from build123d import *

# Parameters (mm, degrees)
SKETCH1_W           = 22
SKETCH1_H           = 112
BOSS_EXTRUDE1_DEPTH = 21
CUT_EXTRUDE1_DEPTH  = 19
FILLET1_START       = -1
FILLET1_DEPTH       = 113
FILLET1_2_DEPTH     = 113
FILLET1_3_DEPTH     = 24
CUT_EXTRUDE11_DEPTH = 116.870617501


with BuildPart() as part:
    # Sketch1 → Boss-Extrude1 (new body)
    with BuildSketch(Plane(origin=(0, 0, 0), x_dir=(1, 0, 0), z_dir=(0, 1, 0))):
        with Locations((11, -56)):
            Rectangle(SKETCH1_W, SKETCH1_H)
    extrude(amount=BOSS_EXTRUDE1_DEPTH)

    # Sketch2 → Cut-Extrude1 (cut)
    with BuildSketch(Plane.XZ):
        Polygon((0, 112), (22, 112), (22, 0), (21, 0), (21, 111), (1, 111), (1, 0), (0, 0), align=None)
    extrude(amount=-CUT_EXTRUDE1_DEPTH, mode=Mode.SUBTRACT)

    # Fillet1: read off the stored shape, not the designer's step
    # Fillet1 outline → Fillet1 (cut)
    with BuildSketch(Plane.XY.offset(FILLET1_START)):
        with BuildLine():
            Line((0, 19), (1, 19))
            ThreePointArc((1, 19), (0.292893219, 19.292893219), (0, 20))
            Line((0, 20), (0, 19))
        make_face()
        with BuildLine():
            ThreePointArc((22, 20), (21.707106781, 19.292893219), (21, 19))
            Line((21, 19), (22, 19))
            Line((22, 19), (22, 20))
        make_face()
    extrude(amount=FILLET1_DEPTH, mode=Mode.SUBTRACT)

    # Fillet1 2 outline → Fillet1 2 (cut)
    with BuildSketch(Plane.XY.offset(FILLET1_START)):
        with BuildLine():
            Line((0, 21), (0, 20))
            ThreePointArc((0, 20), (0.292893219, 20.707106781), (1, 21))
            Line((1, 21), (0, 21))
        make_face()
        with BuildLine():
            Line((22, 21), (21, 21))
            ThreePointArc((21, 21), (21.707106781, 20.707106781), (22, 20))
            Line((22, 20), (22, 21))
        make_face()
    extrude(amount=FILLET1_2_DEPTH, mode=Mode.SUBTRACT)

    # Fillet1 3 outline → Fillet1 3 (cut)
    with BuildSketch(Plane.YZ.offset(FILLET1_START)):
        with BuildLine():
            Line((21, 112), (20, 112))
            ThreePointArc((20, 112), (20.707106781, 111.707106781), (21, 111))
            Line((21, 111), (21, 112))
        make_face()
        with BuildLine():
            ThreePointArc((19, 111), (19.292893219, 111.707106781), (20, 112))
            Line((20, 112), (19, 112))
            Line((19, 112), (19, 111))
        make_face()
    extrude(amount=FILLET1_3_DEPTH, mode=Mode.SUBTRACT)

    # Sketch11 → Cut-Extrude11 (cut, through all)
    with BuildSketch(Plane.ZY.offset(-1)):
        Polygon((0, 0), (111, 0), (111, 7.767718463), align=None)
    extrude(amount=-CUT_EXTRUDE11_DEPTH, mode=Mode.SUBTRACT)


solid = part.part
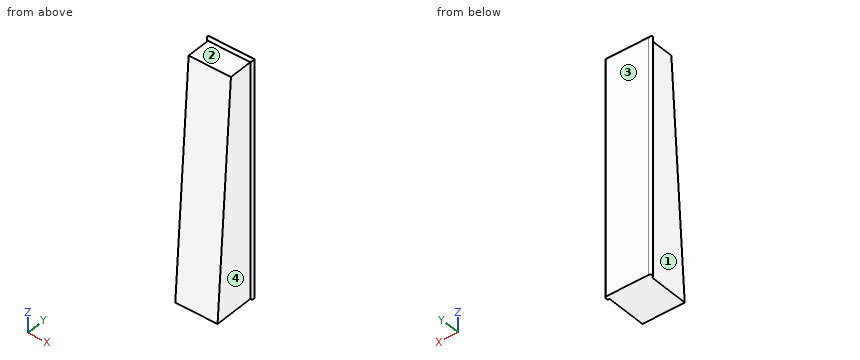
Work out the finished part from the listing and answer in its coordinate system (mm). Face numbers are marked on the shaded views. A direction names the side the tool comes from. Give positions to 0.01 mm unless a question says otherwise; leave off trailing zeros. Order: outer loops, then holes, each group sorted by start corner. A loop starts at its lowest first (then second) coordinate and runs counter-clockwise, first axis right, second up. Notation, with made-up numbers: (34, -22) - (77, -22) arc R16 ccw to (77, 9) - close; hole circle Ø8 at (41.5, 1.25). An arc over 180 degrees is marked (long way). Answer as CSV lines item,"result". Start each with the question number.
Q1. The part is cut by section C-C (y = 16). Write down the section's boundary in (x, z), then the cut area to 3 significant figures.
Q2. The part is cut by section A-A (z = 93). Write down the section's boundary in (x, y), then the cut area to 3 significant figures.
Q3. The part is cut by section B-B (x = 6). Write down the section's boundary in (y, z), then the cut area to 3 significant figures.
Q4. The part is cut by section D-D (z = 36). Write down the section's boundary in (x, y).
Q5. For the marked faces 1, 2, 3 and 4, determine the directions among +Z, -Z, +X, -X, +Y, -Y from which every point of the face is accessible in a straight line to the end or side of a thin tool.
Q6. Given pin 1 Ø8 at (x, z) = (11, 15) entering from -Y; pin 2 Ø9.5 at (y, z) = (12.5, 57) entering from -X; pin 3 Ø5.5 at (y, z) = (11, 48) entering from +X; pin 4 Ø2 at (y, z) = (2, 67) entering from +X, each flat-ended and moving along its own axis, determine where each tip first touches the part or whether it passes through.
Q7. Find the intervals of material crossed by L1, parallel to X at y = 2.75, z = 23; L2, parallel to Z at x = 20.25, y = 11.25; L3, parallel to Y at x = 2.5, z = 84.5, in increasing order. Write a range as [from, to].
Check result:
1,outline,"(1, 0) - (21, 0) - (21, 111) - (1, 111) - close"
1,area,"2,220 mm²"
2,outline,"(1, 6.51) - (21, 6.51) - (21, 19) arc R1 ccw to (21, 21) - (1, 21) arc R1 ccw to (1, 19) - close"
2,area,"293 mm²"
3,outline,"(0, 0) - (21, 0) - (21, 111) arc R1 ccw to (19, 111) - (7.77, 111) - close"
3,area,"1,900 mm²"
4,outline,"(1, 2.52) - (21, 2.52) - (21, 19) arc R1 ccw to (21, 21) - (1, 21) arc R1 ccw to (1, 19) - close"
5,face 1,"+Z, -Z, -X, -Y"
5,face 2,"+Z, +X, -X, -Y"
5,face 3,"+Z, -Z, +X, -X, +Y"
5,face 4,"+Z, -Z, +X, -Y"
6,pin 1,"stops at y = 0.77"
6,pin 2,"stops at x = 1"
6,pin 3,"stops at x = 21"
6,pin 4,"passes through"
7,L1,"x = [1, 21]"
7,L2,"z = [0, 111]"
7,L3,"y = [5.91, 21]"
